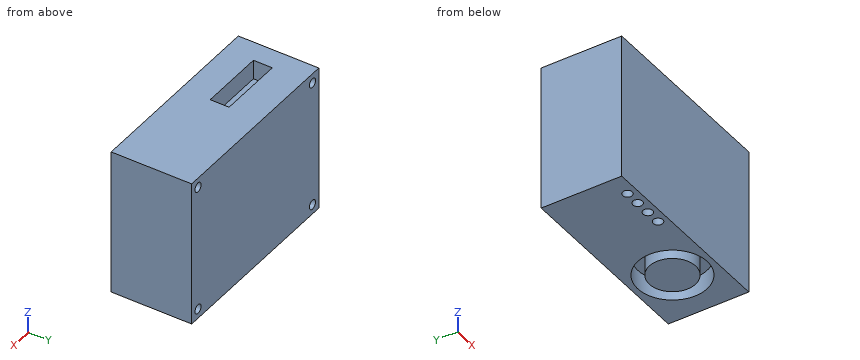
from build123d import *

# Parameters (mm, degrees)
SKETCH1_W                = 50
SKETCH1_H                = 38
BOSS_EXTRUDE1_DEPTH      = 20.9
M2_CLEARANCE_HOLE1_D     = 2.4
M2_CLEARANCE_HOLE1_DEPTH = 10
M2_CLEARANCE_HOLE1_TIP   = 0.721032743
SKETCH5_R                = 9
SKETCH5_R_2              = 6
SKETCH5_R_3              = 1.25
CUT_EXTRUDE1_DEPTH       = 5
SKETCH6_W                = 17
SKETCH6_H                = 4.9
CUT_EXTRUDE2_DEPTH       = 5


with BuildPart() as part:
    # Sketch1 → Boss-Extrude1 (new body)
    with BuildSketch(Plane(origin=(0, 0, 0), x_dir=(1, 0, 0), z_dir=(0, 1, 0))):
        with Locations((-1.258426966, -2.882022472)):
            Rectangle(SKETCH1_W, SKETCH1_H)
    extrude(amount=BOSS_EXTRUDE1_DEPTH)

    # M2 Clearance Hole1
    with Locations(Plane(origin=(0, 20.9, 0), x_dir=(1, 0, 0), z_dir=(0, 1, 0))):
        with Locations((-23.758426966, 13.617977528), (-23.758426966, -19.382022472), (21.241573034, -19.382022472), (21.241573034, 13.617977528)):
            Hole(M2_CLEARANCE_HOLE1_D / 2, depth=M2_CLEARANCE_HOLE1_DEPTH)
            with Locations((0, 0, -(M2_CLEARANCE_HOLE1_DEPTH + M2_CLEARANCE_HOLE1_TIP / 2))):  # 118° drill point
                Cone(0, M2_CLEARANCE_HOLE1_D / 2, M2_CLEARANCE_HOLE1_TIP, mode=Mode.SUBTRACT)

    # Sketch5 → Cut-Extrude1 (cut)
    # profile 1 of 5: a face of its own
    with BuildSketch(Plane(origin=(0, 0, -16.117977528), x_dir=(-1, 0, 0), z_dir=(0, 0, -1))):
        with Locations((-9.541573034, 10.45)):
            Circle(SKETCH5_R)
        with Locations((-9.541573034, 10.45)):
            Circle(SKETCH5_R_2, mode=Mode.SUBTRACT)
    # profile 2 of 5: a face of its own
    with BuildSketch(Plane(origin=(0, 0, -16.117977528), x_dir=(-1, 0, 0), z_dir=(0, 0, -1))):
        with Locations((20.258426966, 2.45)):
            Circle(SKETCH5_R_3)
    # profile 3 of 5: a face of its own
    with BuildSketch(Plane(origin=(0, 0, -16.117977528), x_dir=(-1, 0, 0), z_dir=(0, 0, -1))):
        with Locations((16.258426966, 2.45)):
            Circle(SKETCH5_R_3)
    # profile 4 of 5: a face of its own
    with BuildSketch(Plane(origin=(0, 0, -16.117977528), x_dir=(-1, 0, 0), z_dir=(0, 0, -1))):
        with Locations((12.258426966, 2.45)):
            Circle(SKETCH5_R_3)
    # profile 5 of 5: a face of its own
    with BuildSketch(Plane(origin=(0, 0, -16.117977528), x_dir=(-1, 0, 0), z_dir=(0, 0, -1))):
        with Locations((8.258426966, 2.45)):
            Circle(SKETCH5_R_3)
    extrude(amount=-CUT_EXTRUDE1_DEPTH, mode=Mode.SUBTRACT)

    # Sketch6 → Cut-Extrude2 (cut)
    with BuildSketch(Plane.XY.offset(21.882022472)):
        with Locations((-12.258426966, 10)):
            Rectangle(SKETCH6_W, SKETCH6_H)
    extrude(amount=-CUT_EXTRUDE2_DEPTH, mode=Mode.SUBTRACT)


solid = part.part
CAD build for the part. Positions are in the model's coordinates, mm. Round coordinates to 2 decimals unless told otherwise and drop trailing zeros. Order: outer loops, then holes, each group sorted by start corner. A loop starts at its lowest first (then second) coordinate and runs counter-clockwise, first axis right, second up. Notation, with made-up numbers: (51, -26.75) - (91, -26.75) arc R9 cw to (91, -10.75) - close; hole circle Ø3 at (16.5, 24). An arc over 180 degrees is marked (long way). Return JSON: item names as keys, results as strings.
(1) Cut at C-C (y = 9.25). Give the cut face in (x, z), then the cut area to 3 significant figures.
Answer key:
{"outline": "(-26.26, -16.12) - (0.62, -16.12) - (0.62, -11.12) - (3.66, -11.12) - (3.66, -16.12) - (15.42, -16.12) - (15.42, -11.12) - (18.46, -11.12) - (18.46, -16.12) - (23.74, -16.12) - (23.74, 21.88) - (-3.76, 21.88) - (-3.76, 16.88) - (-20.76, 16.88) - (-20.76, 21.88) - (-26.26, 21.88) - close", "area": "1,780 mm^2"}
(2) Cut at A-A (y = 15). Give the cut face in (x, z).
Answer key:
{"outline": "(-26.26, -16.12) - (1.78, -16.12) - (1.78, -11.12) - (5.63, -11.12) - (5.63, -16.12) - (13.45, -16.12) - (13.45, -11.12) - (17.31, -11.12) - (17.31, -16.12) - (23.74, -16.12) - (23.74, 21.88) - (-26.26, 21.88) - close; hole circle Ø2.4 at (-23.76, -13.62); hole circle Ø2.4 at (-23.76, 19.38); hole circle Ø2.4 at (21.24, -13.62); hole circle Ø2.4 at (21.24, 19.38)"}
(3) Cut at B-B (x = -8.5). Give the cut face in (y, z), then the cut area to 3 significant figures.
Answer key:
{"outline": "(0, -16.12) - (1.22, -16.12) - (1.22, -11.12) - (3.68, -11.12) - (3.68, -16.12) - (20.9, -16.12) - (20.9, 21.88) - (12.45, 21.88) - (12.45, 16.88) - (7.55, 16.88) - (7.55, 21.88) - (0, 21.88) - close", "area": "757 mm^2"}
(4) Pin check, flat tip, straight feed: pin 1 Ø1.5 at (x, y) = (-12.26, 2.45) entering from -Z. Stop position of the tip, or through.
Answer key:
{"pin 1": "stops at z = -11.12"}
(5) Wall check: probe 1 along X at (y, z) = (15.75, -11.5); probe 2 along Z at (x, y) = (-6.5, 8.75); probe 3 along Y at (x, z) = (8.5, -12.5). Give the ranges that are in metal, low to high. Write a range as from..to.
Answer key:
{"probe 1": "x = -26.26..2.27, 6.73..12.35, 16.82..23.74", "probe 2": "z = -16.12..16.88", "probe 3": "y = 0..1.51, 4.54..16.36, 19.39..20.9"}
(6) Cut at D-D (x = 5.5). Give the cut face in (y, z), then the cut area to 3 significant figures.
Answer key:
{"outline": "(0, -16.12) - (2.41, -16.12) - (2.41, -11.12) - (6.02, -11.12) - (6.02, -16.12) - (14.88, -16.12) - (14.88, -11.12) - (18.49, -11.12) - (18.49, -16.12) - (20.9, -16.12) - (20.9, 21.88) - (0, 21.88) - close", "area": "758 mm^2"}
